Here's how the part is built. I have some questions about the finished solid (model axes, mm). Round coordinates to 2 decimals unless told otherwise and drop trailing zeros. Write each loop counter-clockwise with the first axis right and the second up, starting at its lowest first coordinate (ties: lowest second). Pieces come first, ordered by that corner, then holes. Notation, with made-up numbers: M -31.5,79 L -20.5,79 A16 ccw -20.5,97 Z; hole C 71.5,-13.75 d7. An arc over 180 degrees is marked long. Use a Markdown table: item, result. Add a question column.
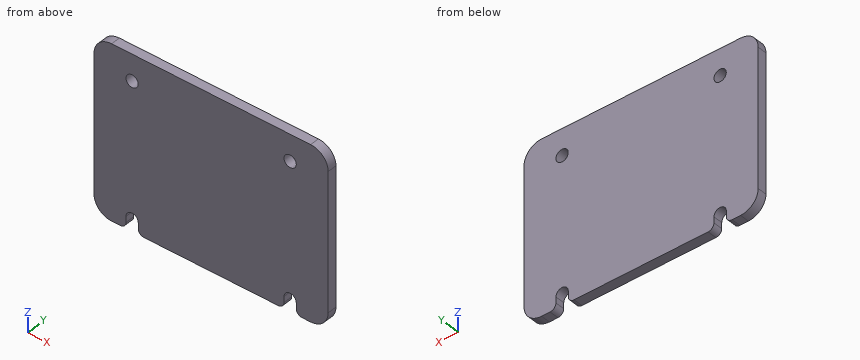
```python
from build123d import *

# Parameters (mm, degrees)
SKETCH1_W                = 40
SKETCH1_H                = 29.5
BOSS_EXTRUDE1_DEPTH      = 1.6
FILLET1_R                = 3
M2_CLEARANCE_HOLE3_D     = 2.1
M2_CLEARANCE_HOLE3_DEPTH = 5.2
M2_CLEARANCE_HOLE3_TIP   = 0.63090365
CUT_EXTRUDE2_DEPTH       = 25.902258934
CUT_EXTRUDE2_DEPTH_BACK  = 25.902258934
FILLET3_R                = 1


with BuildPart() as part:
    # Sketch1 → Boss-Extrude1 (new body)
    with BuildSketch(Plane(origin=(0, 0, 0), x_dir=(1, 0, 0), z_dir=(0, 1, 0))):
        Rectangle(SKETCH1_W, SKETCH1_H)
    extrude(amount=BOSS_EXTRUDE1_DEPTH)

    # Fillet1
    fillet1_edges = [part.edges().sort_by_distance(p)[0] for p in [
        (-20, 0.8, -14.75),
        (20, 0.8, -14.75),
        (20, 0.8, 14.75),
        (-20, 0.8, 14.75),
    ]]
    fillet(fillet1_edges, radius=FILLET1_R)

    # M2 Clearance Hole3
    with Locations(Plane(origin=(0, 1.6, 0), x_dir=(1, 0, 0), z_dir=(0, 1, 0))):
        with Locations((-13.5, 12.75), (13.5, 12.75), (13.5, -10.25), (-13.5, -10.25)):
            Hole(M2_CLEARANCE_HOLE3_D / 2, depth=M2_CLEARANCE_HOLE3_DEPTH)
            with Locations((0, 0, -(M2_CLEARANCE_HOLE3_DEPTH + M2_CLEARANCE_HOLE3_TIP / 2))):  # 118° drill point
                Cone(0, M2_CLEARANCE_HOLE3_D / 2, M2_CLEARANCE_HOLE3_TIP, mode=Mode.SUBTRACT)

    # Sketch10 → Cut-Extrude2 (cut, two sides: drawn at the far end of the back side and taken through both)
    with BuildSketch(Plane(origin=(0, 1.6, 0), x_dir=(1, 0, 0), z_dir=(0, 1, 0)).offset(-CUT_EXTRUDE2_DEPTH_BACK)):
        with BuildLine():
            Line((-14.55, 12.75), (-14.55, 17.75))
            ThreePointArc((-14.55, 17.75), (-13.5, 18.8), (-12.45, 17.75))
            Line((-12.45, 17.75), (-12.45, 12.75))
            ThreePointArc((-12.45, 12.75), (-13.5, 11.7), (-14.55, 12.75))
        make_face()
        with BuildLine():
            Line((14.55, 12.75), (14.55, 17.75))
            ThreePointArc((14.55, 17.75), (13.5, 18.8), (12.45, 17.75))
            Line((12.45, 17.75), (12.45, 12.75))
            ThreePointArc((12.45, 12.75), (13.5, 11.7), (14.55, 12.75))
        make_face()
    extrude(amount=CUT_EXTRUDE2_DEPTH + CUT_EXTRUDE2_DEPTH_BACK, mode=Mode.SUBTRACT)

    # Fillet3
    fillet3_edges = [part.edges().sort_by_distance(p)[0] for p in [
        (-14.55, 0.8, -14.75),
        (-12.45, 0.8, -14.75),
        (12.45, 0.8, -14.75),
        (14.55, 0.8, -14.75),
    ]]
    fillet(fillet3_edges, radius=FILLET3_R)


solid = part.part
```
Item 1: For pin 1 Ø0.5 at (y, z) = (0.5, -13.5) entering from +X; pin 2 Ø1.3 at (x, z) = (-13.5, 10.25) entering from -Y, each with a flat end and sliding along its axis, tell me the tip position at first contact or that it passes through.
Item 2: Imagine slicing it at A-A on x = -13.5. List the corners of the cut face in (y, z) for me, plus the area to 3 significant figures.
Item 3: I need wall thicknesses on probe 1 along X at (y, z) = (1.2, 10.25); probe 2 along Z at (x, y) = (-13.5, 1.3); probe 3 along Z at (x, y) = (-13, 0.3). Which ranges of each line are inside material? Lowest first, please. Write a range as from..to.
Item 4: Imagine slicing it at B-B on y = 0.45. List the corners of the cut face in (x, z) for me, plus the area to 3 significant figures.
The answers:
| question | item | result |
|---|---|---|
| 1 | pin 1 | x = 19.6 |
| 1 | pin 2 | through |
| 2 | outline | M 0,-11.7 L 1.6,-11.7 L 1.6,9.2 L 0,9.2 Z; M 0,11.3 L 1.6,11.3 L 1.6,14.75 L 0,14.75 Z |
| 2 | area | 39.0 mm² |
| 3 | probe 1 | -20..-14.55, -12.45..12.45, 14.55..20 |
| 3 | probe 2 | -11.7..9.2, 11.3..14.75 |
| 3 | probe 3 | -11.83..9.33, 11.17..14.75 |
| 4 | outline | M -20,-11.75 A3 ccw -17,-14.75 L -15.55,-14.75 A1 ccw -14.55,-13.75 L -14.55,-12.75 A1.05 cw -12.45,-12.75 L -12.45,-13.75 A1 ccw -11.45,-14.75 L 11.45,-14.75 A1 ccw 12.45,-13.75 L 12.45,-12.75 A1.05 cw 14.55,-12.75 L 14.55,-13.75 A1 ccw 15.55,-14.75 L 17,-14.75 A3 ccw 20,-11.75 L 20,11.75 A3 ccw 17,14.75 L -17,14.75 A3 ccw -20,11.75 Z; hole C -13.5,10.25 d2.1; hole C 13.5,10.25 d2.1 |
| 4 | area | 1,150 mm² |
